The model under review builds one solid part; all positions refer to its coordinate system, in mm. Coordinates: 2 decimals unless noted, no trailing zeros. Loops run counter-clockwise (first coordinate to the right, second up) from the corner with the lowest first, then second, coordinate; pieces in that order, holes last. Notation, with made-up numbers: M -8,17 L 33,17 A14 cw 33,22 Z; hole C 39,-33.75 d1. An arc over 180 degrees is marked long. Use CSV: the item, a comma, the result in double quotes. Start each with the question number.
1. Clearance check with flat-ended pins moving along their axes: P1, Ø0.5, axis at x = 29.5, z = 0.5, coming from the -Y side; P2, Ø0.5, axis at x = 22, z = 0.5, coming from the +Y side. State where each tip first meets the part, or that it passes through.
2. For L1, parallel to Y at x = 6, z = 0.6; L2, parallel to Y at x = 5, z = 0.8; L3, parallel to X at y = 17, z = 0.75, list the stretches that pass through material, from the lowest coordinate up.
3. Add section A-A, the plane y = 29.25. Write out the cut boundary in (x, z).
4. Add section B-B, the plane x = 33.5. Write out the cut boundary in (y, z), then the cut area to 3 significant figures.
5. Add section D-D, the plane z = 0.7. State how many separate pieces and enclosed holes the cut face has, then the cut area to 3 significant figures.
6. Add section C-C, the plane x = 6. Write out the cut boundary in (y, z), then the cut area to 3 significant figures.
from build123d import *

# Parameters (mm, degrees)
SKETCH1_W           = 45
SKETCH1_H           = 103
BOSS_EXTRUDE1_DEPTH = 1
FILLET1_R           = 8
SKETCH2_R           = 4
CUT_EXTRUDE1_DEPTH  = 1
CUT_EXTRUDE2_DEPTH  = 1
BOSS_EXTRUDE2_DEPTH = 1
SKETCH5_R           = 7.5
CUT_EXTRUDE3_DEPTH  = 10
FILLET2_R           = 3


with BuildPart() as part:
    # Sketch1 → Boss-Extrude1 (new body)
    with BuildSketch(Plane.XY):
        with Locations((22.5, 51.5)):
            Rectangle(SKETCH1_W, SKETCH1_H)
        with BuildLine():
            Line((10.75, 22.25), (34.25, 22.25))
            ThreePointArc((34.25, 22.25), (41.5, 15), (34.25, 7.75))
            Line((34.25, 7.75), (10.75, 7.75))
            ThreePointArc((10.75, 7.75), (3.5, 15), (10.75, 22.25))
        make_face(mode=Mode.SUBTRACT)
    extrude(amount=BOSS_EXTRUDE1_DEPTH)

    # Fillet1
    fillet1_edges = [part.edges().sort_by_distance(p)[0] for p in [
        (0, 103, 0.5),
        (45, 103, 0.5),
        (45, 0, 0.5),
        (0, 0, 0.5),
    ]]
    fillet(fillet1_edges, radius=FILLET1_R)

    # Sketch2 → Cut-Extrude1 (cut)
    with BuildSketch(Plane.XY.offset(1)):
        with Locations((6, 29.25)):
            Circle(SKETCH2_R)
    extrude(amount=-CUT_EXTRUDE1_DEPTH, mode=Mode.SUBTRACT)

    # Sketch3 → Cut-Extrude2 (cut)
    with BuildSketch(Plane.XY.offset(1)):
        Polygon((17, 98.5), (28, 98.5), (36, 103), (9, 103), align=None)
        Polygon((17, 4.5), (28, 4.5), (36, 0), (9, 0), align=None)
    extrude(amount=-CUT_EXTRUDE2_DEPTH, mode=Mode.SUBTRACT)

    # Sketch4 → Boss-Extrude2 (add)
    with BuildSketch(Plane.XY.offset(1)):
        with BuildLine():
            Line((9.607201991, 23.81242846), (35.392798009, 23.81242846))
            ThreePointArc((35.392798009, 23.81242846), (44.205226468, 15), (35.392798009, 6.18757154))
            Line((35.392798009, 6.18757154), (9.607201991, 6.18757154))
            ThreePointArc((9.607201991, 6.18757154), (0.794773532, 15), (9.607201991, 23.81242846))
        make_face()
        with BuildLine():
            Line((10, 21.25), (18.354219012, 21.25))
            ThreePointArc((18.354219012, 21.25), (22.5, 22.5), (26.645780988, 21.25))
            Line((26.645780988, 21.25), (35, 21.25))
            ThreePointArc((35, 21.25), (41.25, 15), (35, 8.75))
            Line((35, 8.75), (26.645780988, 8.75))
            ThreePointArc((26.645780988, 8.75), (22.5, 7.5), (18.354219012, 8.75))
            Line((18.354219012, 8.75), (10, 8.75))
            ThreePointArc((10, 8.75), (3.75, 15), (10, 21.25))
        make_face(mode=Mode.SUBTRACT)
    extrude(amount=-BOSS_EXTRUDE2_DEPTH)

    # Sketch5 → Cut-Extrude3 (cut)
    with BuildSketch(Plane.XY.offset(1)):
        with Locations((22.5, 15)):
            Circle(SKETCH5_R)
    extrude(amount=-CUT_EXTRUDE3_DEPTH, mode=Mode.SUBTRACT)

    # Fillet2
    fillet2_edges = [part.edges().sort_by_distance(p)[0] for p in [
        (36, 103, 0.5),
        (28, 98.5, 0.5),
        (17, 98.5, 0.5),
        (9, 103, 0.5),
        (28, 4.5, 0.5),
        (36, 0, 0.5),
        (9, 0, 0.5),
        (17, 4.5, 0.5),
    ]]
    fillet(fillet2_edges, radius=FILLET2_R)


solid = part.part
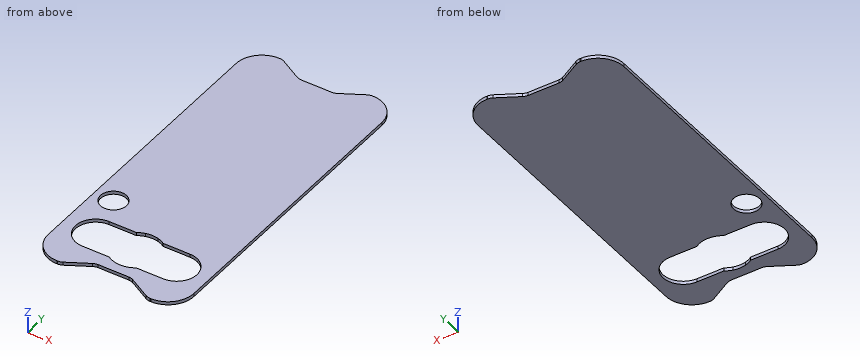
Computed:
1,P1,"stops at y = 3.52"
1,P2,"stops at y = 98.5"
2,L1,"y = 0.25 to 10.2, 19.8 to 25.25, 33.25 to 102.75"
2,L2,"y = 0.58 to 11.25, 18.75 to 25.38, 33.12 to 102.42"
2,L3,"x = 0 to 4.08, 40.92 to 45"
3,outline,"M 0,0 L 2,0 L 2,1 L 0,1 Z; M 10,0 L 45,0 L 45,1 L 10,1 Z"
4,outline,"M 1.41,0 L 8.75,0 L 8.75,1 L 1.41,1 Z; M 21.25,0 L 101.59,0 L 101.59,1 L 21.25,1 Z"
4,area,"87.7 mm^2"
5,separate pieces,"1"
5,enclosed holes,"2"
5,area,"3,910 mm^2"
6,outline,"M 0.25,0 L 10.2,0 L 10.2,1 L 0.25,1 Z; M 19.8,0 L 25.25,0 L 25.25,1 L 19.8,1 Z; M 33.25,0 L 102.75,0 L 102.75,1 L 33.25,1 Z"
6,area,"84.9 mm^2"
